Could you check a few things on this model? Use its own coordinates, in mm. A direction names the side the tool comes from. Give positions to 0.01 mm unless a question says otherwise; leave off trailing zeros. Order: outer loops, then holes, each group sorted by start corner. A loop starts at its lowest first (then second) coordinate and runs counter-clockwise, first axis right, second up.
from build123d import *

# Parameters (mm, degrees)
F0_W          = 26.5
F0_H          = 33.5
F1_DEPTH      = 25
F2_W          = 16.5
F2_H          = 23.5
F3_DEPTH      = 20
F4_R          = 2.5
F5_DEPTH      = 25.001
F7_DEPTH      = 31
F7_DEPTH_BACK = 35
F8_R          = 2
F10_DEPTH     = 5


# Not quite as in the source:
# - a feature names something its author has since deleted; it is built from what else it names


with BuildPart() as f1:
    # F0 (on Right) → F1 (new body)
    with BuildSketch(Plane.YZ):
        with Locations((8.25, 11.75)):
            Rectangle(F0_W, F0_H)
    extrude(amount=F1_DEPTH)

    # F2 (on face) → F3 (cut)
    with BuildSketch(Plane.YZ.offset(25)):
        with Locations((8.25, 11.75)):
            Rectangle(F2_W, F2_H)
    extrude(amount=-F3_DEPTH, mode=Mode.SUBTRACT)

    # F4 (on face) → F5 (cut, through all)
    with BuildSketch(Plane(origin=(0, 0, 0), x_dir=(0, -1, 0), z_dir=(-1, 0, 0))):
        with Locations((-8.25, 11.75)):
            Circle(F4_R)
    extrude(amount=-F5_DEPTH, mode=Mode.SUBTRACT)

    # F6 (on face) → F7 (join, two sides)
    with BuildSketch(Plane.YZ.offset(25)) as f7_sk:
        Polygon((-5, -5), (-14.75, -5), (-14.75, -10), (30.18, -10), (30.18, -5), (21.5, -5), align=None)
    extrude(amount=F7_DEPTH)
    extrude(f7_sk.sketch, amount=-F7_DEPTH_BACK)

    # F8
    f8_edges = [f1.edges().sort_by_distance(p)[0] for p in [
        (56, -14.75, -7.5),
        (56, 30.18, -7.5),
        (-10, -14.75, -7.5),
        (-10, 30.18, -7.5),
    ]]
    fillet(f8_edges, radius=F8_R)

    # F9 (on face) → F10 (cut, through all)
    with BuildSketch(Plane.XY.offset(-5)):
        with BuildLine():
            ThreePointArc((30.47, 21.46), (28.702233047, 20.727766953), (27.97, 18.96))
            Line((27.97, 18.96), (27.97, 11.96))
            ThreePointArc((27.97, 11.96), (28.702233047, 10.192233047), (30.47, 9.46))
            ThreePointArc((30.47, 9.46), (32.237766953, 10.192233047), (32.97, 11.96))
            Line((32.97, 11.96), (32.97, 18.96))
            ThreePointArc((32.97, 18.96), (32.237766953, 20.727766953), (30.47, 21.46))
        make_face()
        with BuildLine():
            ThreePointArc((30.47, 1.25), (28.702233047, 0.517766953), (27.97, -1.25))
            Line((27.97, -1.25), (27.97, -8.25))
            ThreePointArc((27.97, -8.25), (28.702233047, -10.017766953), (30.47, -10.75))
            ThreePointArc((30.47, -10.75), (32.237766953, -10.017766953), (32.97, -8.25))
            Line((32.97, -8.25), (32.97, -1.25))
            ThreePointArc((32.97, -1.25), (32.237766953, 0.517766953), (30.47, 1.25))
        make_face()
        with BuildLine():
            ThreePointArc((48.4, 21.46), (46.632233047, 20.727766953), (45.9, 18.96))
            Line((45.9, 18.96), (45.9, 11.96))
            ThreePointArc((45.9, 11.96), (46.632233047, 10.192233047), (48.4, 9.46))
            ThreePointArc((48.4, 9.46), (50.167766953, 10.192233047), (50.9, 11.96))
            Line((50.9, 11.96), (50.9, 18.96))
            ThreePointArc((50.9, 18.96), (50.167766953, 20.727766953), (48.4, 21.46))
        make_face()
        with BuildLine():
            ThreePointArc((48.4, 1.25), (46.632233047, 0.517766953), (45.9, -1.25))
            Line((45.9, -1.25), (45.9, -8.25))
            ThreePointArc((45.9, -8.25), (46.632233047, -10.017766953), (48.4, -10.75))
            ThreePointArc((48.4, -10.75), (50.167766953, -10.017766953), (50.9, -8.25))
            Line((50.9, -8.25), (50.9, -1.25))
            ThreePointArc((50.9, -1.25), (50.167766953, 0.517766953), (48.4, 1.25))
        make_face()
        with BuildLine():
            ThreePointArc((-5, 14.25), (-6.767766953, 13.517766953), (-7.5, 11.75))
            Line((-7.5, 11.75), (-7.5, 4.75))
            ThreePointArc((-7.5, 4.75), (-6.767766953, 2.982233047), (-5, 2.25))
            ThreePointArc((-5, 2.25), (-3.232233047, 2.982233047), (-2.5, 4.75))
            Line((-2.5, 4.75), (-2.5, 11.75))
            ThreePointArc((-2.5, 11.75), (-3.232233047, 13.517766953), (-5, 14.25))
        make_face()
    extrude(amount=-F10_DEPTH, mode=Mode.SUBTRACT)


solid = f1.part
Item 1: Imagine slicing it at B-B on y = 8.25. List the corners of the cut face in (x, z) for me, then the cut area to 4 significant figures.
Findings:
outline: (-10, -10) - (-7.5, -10) - (-7.5, -5) - (-10, -5) - close; (-2.5, -10) - (56, -10) - (56, -5) - (25, -5) - (25, 0) - (5, 0) - (5, 9.25) - (0, 9.25) - (0, -5) - (-2.5, -5) - close; (0, 14.25) - (5, 14.25) - (5, 23.5) - (25, 23.5) - (25, 28.5) - (0, 28.5) - close
area: 647.5 mm2
Item 2: Imagine slicing it at C-C on z = 1.5. List the corners of the cut face in (x, y) for me, then the cut area to 4 significant figures.
Findings:
outline: (0, -5) - (25, -5) - (25, 0) - (5, 0) - (5, 16.5) - (25, 16.5) - (25, 21.5) - (0, 21.5) - close
area: 332.5 mm2
Item 3: We'd pull the mould along X, two halves only. Please class faces 1 (the cylindrical face through (-9.4, -14.18, -7.54)), 2 (the flat face through (5, 8, 15)), 3 (the flat face through (32.97, 15, -7)): +X half, -X half, draft (parallel to the pull), parting line (faces both ways), or undercut.
Findings:
face 1: -X half
face 2: +X half
face 3: undercut
Item 4: For pin 1 (5 mm diameter, centred on x = 36.5, y = -7.5, fed in from +Z); pin 2 (13 mm diameter, centred on y = 9, z = 14.5, fed in from -X); pin 3 (8 mm diameter, centred on y = 8.5, z = 5, fed in from +X), each with a flat end and sliding along its axis, tell me the tip position at first contact or that it passes through.
Findings:
pin 1: stops at z = -5
pin 2: stops at x = 0
pin 3: stops at x = 5
Item 5: Please list where these lines run through material, in increasing order: line 1 along Z through (x, y) = (3, 8); line 2 along Z through (x, y) = (26, -8); line 3 along Y through (x, z) = (19.5, 4.5).
Findings:
line 1: z = -10 to 9.26, 14.24 to 28.5
line 2: z = -10 to -5
line 3: y = -5 to 0, 16.5 to 21.5
Item 6: Imagine slicing it at D-D on x = -4. List the corners of the cut face in (y, z) for me.
Findings:
outline: (-14.75, -10) - (2.46, -10) - (2.46, -5) - (-14.75, -5) - close; (14.04, -10) - (30.18, -10) - (30.18, -5) - (14.04, -5) - close
Item 7: For faces 4 (the flat face through (45.9, -5, -7)), 5 (the flat face through (15, 8, 23.5)), 6 (the flat face through (12, 21.5, 12)), which set-ups out of +Z, -Z, +X, -X, +Y, -Y let a thin tool reach every point of the face, with its end or its side?
Findings:
face 4: +Z, -Z
face 5: +X
face 6: +Z, +X, -X, +Y
Item 8: Imagine slicing it at A-A on z = 11.75. List the corners of the cut face in (x, y) for me.
Findings:
outline: (0, -5) - (25, -5) - (25, 0) - (5, 0) - (5, 5.75) - (0, 5.75) - close; (0, 10.75) - (5, 10.75) - (5, 16.5) - (25, 16.5) - (25, 21.5) - (0, 21.5) - close
